Verification items for the finished model (mm, model axes). Give positions to 0.01 mm unless a question says otherwise; leave off trailing zeros. Write each loop counter-clockwise with the first axis right and the second up, starting at its lowest first coordinate (ties: lowest second). Pieces come first, ordered by that corner, then holes. Notation, with made-up numbers: (-10.75, -0.75) -> (34.25, -0.75) arc R19 cw to (34.25, 9.25) -> close; hole circle Ø11 at (69, 0.5). An arc over 180 degrees is marked (long way). Use one line per item in the form item = value. Start each with the question number.
(1) Release check for a two-part mould opening along Z. For faces 1 (the face through (7.89, -1.08, 4.88)), 2 (the face through (16, -4, -1)), 3 (the face through (8.108, 3.233, -1.341)) record: pulls with the +Z half, pulls with the -Z half, needs draft (parallel to the pull), parting line crosses it, or undercut.
(2) Section check A-A, the plane z = 0. Record the cut outline in (x, y), plus the area to 3 significant figures.
(3) Scan lines: L1, parallel to Z at x = 14, y = 0; L2, parallel to Z at x = 10.75, y = -2.25; L3, parallel to Y at x = 12.75, z = -2.5. Record each from-to range of solid material in increasing order.
(4) Depth check by flat-ended pin: pin 1 Ø3 at (x, y) = (6, 4) entering from +Z. Enter the tip coordinate at first touch or a pass-through.
(5) Section check C-C, the plane x = 9.5. Record the cut outline in (y, z).
Autodesk Inventor part; units mm, degrees
ref_plane "YZ Plane" through (0, 0, 0) normal (1, 0, 0) x (0, 1, 0)
ref_plane "XZ Plane" through (0, 0, 0) normal (0, 1, 0) x (-1, 0, 0)
ref_plane "XY Plane" through (0, 0, 0) normal (0, 0, 1) x (1, 0, 0)
sketch "Sketch_1" plane through (0, 0, 0) normal (0, 0, 1) x (1, 0, 0)
  line L0 (50, 0) -> (-50, 0)
  line L1 (0, 4.85) -> (0, 3.8)
  arc A0 (0, 3.8) -> (0.3, 3.5) centre (0.3, 3.8) ccw
  line L2 (0.3, 3.5) -> (15.7, 3.5)
  arc A1 (15.7, 3.5) -> (16, 3.8) centre (15.7, 3.8) ccw
  line L3 (16, 3.8) -> (16, 4.85)
  line L4 (16, 4.85) -> (15.7, 5)
  line L5 (15.7, 5) -> (0.3, 5)
  line L6 (0.3, 5) -> (0, 4.85)
revolve "Revolution1" add sketch "Sketch_1" angle 360 about axis through (50, 0, 0) along (1, 0, 0)
properties part number "SKF_IR 7X10X16"
Completed:
q1.face_1 = parting line crosses it
q1.face_2 = needs draft
q1.face_3 = undercut
q2.outline = (0, -4.85) -> (0.3, -5) -> (15.7, -5) -> (16, -4.85) -> (16, -3.8) arc R0.3 ccw to (15.7, -3.5) -> (0.3, -3.5) arc R0.3 ccw to (0, -3.8) -> close; (0, 3.8) arc R0.3 ccw to (0.3, 3.5) -> (15.7, 3.5) arc R0.3 ccw to (16, 3.8) -> (16, 4.85) -> (15.7, 5) -> (0.3, 5) -> (0, 4.85) -> close
q2.area = 47.8 mm²
q3.L1 = -5 to -3.5, 3.5 to 5
q3.L2 = -4.47 to -2.68, 2.68 to 4.47
q3.L3 = -4.33 to -2.45, 2.45 to 4.33
q4.pin_1 = 4.33
q5.outline = circle Ø10 at (0, 0); hole circle Ø7 at (0, 0)
